from build123d import *

# Parameters (mm, degrees)
F0_W     = 177.8
F0_H     = 177.8
F1_DEPTH = 6.35
F3_DEPTH = 177.801
F4_W     = 177.8
F4_H     = 1.5875
F5_DEPTH = 1


with BuildPart() as f1:
    # F0 (on Front) → F1 (new body)
    with BuildSketch(Plane.XZ):
        with Locations((88.9, -88.9)):
            Rectangle(F0_W, F0_H)
    extrude(amount=F1_DEPTH)

    # F2 (on face) → F3 (cut, through all)
    with BuildSketch(Plane(origin=(0, 0, 0), x_dir=(0, -1, 0), z_dir=(-1, 0, 0))):
        Polygon((0, -6.35), (6.35, 0), (0, 0), align=None)
    extrude(amount=-F3_DEPTH, mode=Mode.SUBTRACT)

    # F4 (on face) → F5 (cut)
    with BuildSketch(Plane.XZ.offset(6.35)):
        with Locations((88.9, -25.4)):
            Rectangle(F4_W, F4_H)
        with Locations((88.9, -50.8)):
            Rectangle(F4_W, F4_H)
        with Locations((88.9, -76.2)):
            Rectangle(F4_W, F4_H)
        with Locations((88.9, -101.6)):
            Rectangle(F4_W, F4_H)
        with Locations((88.9, -127)):
            Rectangle(F4_W, F4_H)
        with Locations((88.9, -152.4)):
            Rectangle(F4_W, F4_H)
    extrude(amount=-F5_DEPTH, mode=Mode.SUBTRACT)


solid = f1.part
Part model, mm, in its own coordinate system. Give positions to 0.01 mm unless a question says otherwise; leave off trailing zeros. Write each loop counter-clockwise with the first axis right and the second up, starting at its lowest first coordinate (ties: lowest second). Pieces come first, ordered by that corner, then holes.
1) Probe L1, parallel to Z at x = 17, y = -1.25; L2, parallel to Z at x = 100, y = -1.5. List the from-to ranges inside material, lowest first.
Resolved:
L1: z = -177.8 to -5.1
L2: z = -177.8 to -4.85
2) Cut at A-A on x = 90.5. Write the cut outline in (y, z), then the cut area to 3 significant figures.
Resolved:
outline: (-6.35, -177.8) - (0, -177.8) - (0, -6.35) - (-6.35, 0) - (-6.35, -24.61) - (-5.35, -24.61) - (-5.35, -26.19) - (-6.35, -26.19) - (-6.35, -50.01) - (-5.35, -50.01) - (-5.35, -51.59) - (-6.35, -51.59) - (-6.35, -75.41) - (-5.35, -75.41) - (-5.35, -76.99) - (-6.35, -76.99) - (-6.35, -100.81) - (-5.35, -100.81) - (-5.35, -102.39) - (-6.35, -102.39) - (-6.35, -126.21) - (-5.35, -126.21) - (-5.35, -127.79) - (-6.35, -127.79) - (-6.35, -151.61) - (-5.35, -151.61) - (-5.35, -153.19) - (-6.35, -153.19) - close
area: 1,100 mm2
3) Cut at B-B on y = -3.5. Write the cut outline in (x, z), then the cut area to 3 significant figures.
Resolved:
outline: (0, -177.8) - (177.8, -177.8) - (177.8, -2.85) - (0, -2.85) - close
area: 31,100 mm2
4) Pin check, flat tips, straight feed: pin 1 (0.5 mm diameter, centred on x = 48.5, z = -51, fed in from -Y); pin 2 (0.8 mm diameter, centred on x = 51, y = -5.5, fed in from +Z); pin 3 (0.5 mm diameter, centred on x = 132, y = -6, fed in from +Z). Stop position of each tip, or through.
Resolved:
pin 1: stops at y = -5.35
pin 2: stops at z = -0.45
pin 3: stops at z = -0.1
